```python
from build123d import *

# Parameters (mm, degrees)
SKETCH1_R           = 7.65
BOSS_EXTRUDE1_DEPTH = 11.7


with BuildPart() as part:
    # Sketch1 → Boss-Extrude1 (new body)
    with BuildSketch(Plane(origin=(0, 0, 0), x_dir=(1, 0, 0), z_dir=(0, 1, 0))):
        with BuildLine():
            Line((-14.29, 5.977959518), (-14.29, -18.894))
            Line((-14.29, -18.894), (-8.574, -24.61))
            Line((-8.574, -24.61), (8.574, -24.61))
            Line((8.574, -24.61), (14.29, -18.894))
            Line((14.29, -18.894), (14.29, 5.977959518))
            ThreePointArc((14.29, 5.977959518), (9.48764436, 12.244374402), (2.220630541, 15.33))
            Line((2.220630541, 15.33), (-2.220630541, 15.33))
            ThreePointArc((-2.220630541, 15.33), (-9.48764436, 12.244374402), (-14.29, 5.977959518))
        make_face()
        with Locations(Location((0, 0, 0), (0, 0, 270))):
            Circle(SKETCH1_R, mode=Mode.SUBTRACT)
    extrude(amount=BOSS_EXTRUDE1_DEPTH)


solid = part.part
```
Design review of the part built by this model. Coordinates are the model's own, in mm. Give positions to 0.01 mm unless a question says otherwise; leave off trailing zeros. Loops run counter-clockwise (first coordinate to the right, second up) from the corner with the lowest first, then second, coordinate; pieces in that order, holes last. Notation, with made-up numbers: M -39.5,-28 L -7.5,-28 A11 cw -7.5,-9 Z; hole C -23.5,-4 d11. An arc over 180 degrees is marked long. Return JSON: item names as keys, results as strings. Group by question number.
Item 1: Mouldability with a two-part tool opening along X and no side actions: class faces 1 (the flat face through (14.29, 6, 7)), 2 (the cylindrical face through (-9.4, 5.77, -12.31)), 3 (the cylindrical face through (-4.655, 5.768, -6.071)) as released by +X, released by -X, zero draft, split by the parting line, or undercut.
Item 2: Insertion check: pin 1 Ø1.5 at (y, z) = (7, -8.5) entering from -X; pin 2 Ø2 at (y, z) = (10, -8) entering from -X. Each pin has a flat end and moves straight along its axis. Give the tip position at first contact, or say it passes through.
Item 3: We need section B-B (z = 0). Give the boundary of the cut face in (x, y), and give its area (3 significant figures).
Item 4: We need section A-A (x = 0). Give the boundary of the cut face in (y, z), and give its area (3 significant figures).
Item 5: We need section D-D (x = 10.5). Give the boundary of the cut face in (y, z), and give its area (3 significant figures).
Item 6: We need section C-C (y = 7.5). Give the boundary of the cut face in (x, z).
Item 7: For probe 1 along X at (y, z) = (8.75, 0); probe 2 along X at (y, z) = (2.5, 6.5); probe 3 along Z at (x, y) = (-1, 3.75), list the stretches that pass through material, from the lowest coordinate up.
Output:
{
 "1": {"face 1": "released by +X", "face 2": "released by -X", "face 3": "undercut"},
 "2": {"pin 1": "stops at x = -13.41", "pin 2": "stops at x = -13.82"},
 "3": {"outline": "M -14.29,0 L -7.65,0 L -7.65,11.7 L -14.29,11.7 Z; M 7.65,0 L 14.29,0 L 14.29,11.7 L 7.65,11.7 Z", "area": "155 mm^2"},
 "4": {"outline": "M 0,-15.33 L 11.7,-15.33 L 11.7,-7.65 L 0,-7.65 Z; M 0,7.65 L 11.7,7.65 L 11.7,24.61 L 0,24.61 Z", "area": "288 mm^2"},
 "5": {"outline": "M 0,-11.39 L 11.7,-11.39 L 11.7,22.68 L 0,22.68 Z", "area": "399 mm^2"},
 "6": {"outline": "M -14.29,-5.98 A15.49 ccw -2.22,-15.33 L 2.22,-15.33 A15.49 ccw 14.29,-5.98 L 14.29,18.89 L 8.57,24.61 L -8.57,24.61 L -14.29,18.89 Z; hole C 0,0 d15.3"},
 "7": {"probe 1": "x = -14.29 to -7.65, 7.65 to 14.29", "probe 2": "x = -14.29 to -4.03, 4.03 to 14.29", "probe 3": "z = -15.33 to -7.58, 7.58 to 24.61"}
}
